Build history of the part. All positions in model axes, mm. Round coordinates to 2 decimals unless told otherwise and drop trailing zeros. Order: outer loops, then holes, each group sorted by start corner. A loop starts at its lowest first (then second) coordinate and runs counter-clockwise, first axis right, second up. Notation, with made-up numbers: (-31, 3.25) -> (6, 3.25) arc R17 cw to (6, 19.25) -> close; hole circle Ø9 at (-29, -4.5). An arc over 180 degrees is marked (long way). Answer as CSV lines item,"result". Start each with the question number.
```python
from build123d import *

# Parameters (mm, degrees)
F0_R     = 2.16
F1_DEPTH = 1.09
F3_DEPTH = 25
F4_R     = 0.84
F5_DEPTH = 11


with BuildPart() as f1:
    # F0 (on Front) → F1 (new body)
    with BuildSketch(Plane.XZ):
        Circle(F0_R)
    extrude(amount=F1_DEPTH)

    # F2 (on face) → F3 (cut)
    with BuildSketch(Plane.XZ.offset(1.09)):
        with BuildLine():
            ThreePointArc((0.3967272328, 2.1232539892), (-0.0627415539, 2.1590885803), (-0.5193541089, 2.0966333274))
            Line((-0.5193541089, 2.0966333274), (0.3967272328, 2.1232539892))
        make_face()
    extrude(amount=-F3_DEPTH, mode=Mode.SUBTRACT)

    # F4 (on face) → F5 (join)
    with BuildSketch(Plane(origin=(-0.061313438, 0, 2.1099436583), x_dir=(0.9995780464, 0, 0.0290470157), z_dir=(-0.0290470157, 0, 0.9995780464))):
        with Locations((0, -0.5952777421)):
            Circle(F4_R)
    extrude(amount=F5_DEPTH)

    # F6 (on face) → F7 (revolve)
    with BuildSketch(Plane(origin=(-0.3808306108, 0, 13.1053021689), x_dir=(0.9995780464, 0, 0.0290470157), z_dir=(-0.0290470157, 0, 0.9995780464))):
        with BuildLine():
            Line((0, 0.2447222579), (0, 0.7597222579))
            ThreePointArc((0, 0.7597222579), (-1.355, -0.5952777421), (0, -1.9502777421))
            Line((0, -1.9502777421), (0, -1.4352777421))
            ThreePointArc((0, -1.4352777421), (-0.84, -0.5952777421), (0, 0.2447222579))
        make_face()
    revolve(axis=Axis((-0.3808306108, -0.5952777421, 13.1053021689), (0, -1, 0)))


solid = f1.part
```
Q1. Slice it at B-B, the plane x = 1.15. Write the cut outline in (y, z).
Q2. Flat gauge pins, fed straight in: pin 1 Ø1.3 at (x, z) = (0.5, -0.5) entering from -Y; pin 2 Ø1.5 at (x, y) = (0.5, -0.5) entering from +Z; pin 3 Ø1 at (x, y) = (0.5, -1) entering from +Z. Where does each tip first touch, or does it go through?
Q3. Probe L1, parallel to Y at x = -0.6, z = 1.25; L2, parallel to Y at x = 0.1, z = 10.5; L3, parallel to Z at x = 0.1, y = -1.2. List the from-to ranges inside material, lowest first.
Q4. Slice it at A-A, the plane z = 0. Write the cut outline in (x, y), plus the area to 3 significant figures.
Q5. Two-plate mould, pull along Z, no slides. Class faces 1 (the face through (0.597, -0.343, 7.03)), 2 (the face through (0, 0, 0)): +Z half, -Z half, draft (parallel to the pull), parting line (faces both ways), or undercut.
Solutions:
1,outline,"(-1.09, -1.83) -> (0, -1.83) -> (0, 1.83) -> (-1.09, 1.83) -> close"
2,pin 1,"stops at y = -1.09"
2,pin 2,"stops at z = 14.45"
2,pin 3,"stops at z = 14.38"
3,L1,"y = -1.09 to 0"
3,L2,"y = -1.33 to 0.14"
3,L3,"z = 2.11 to 13.12, 13.44 to 14.22"
4,outline,"(-2.16, -1.09) -> (2.16, -1.09) -> (2.16, 0) -> (-2.16, 0) -> close"
4,area,"4.71 mm2"
5,face 1,"undercut"
5,face 2,"draft"
